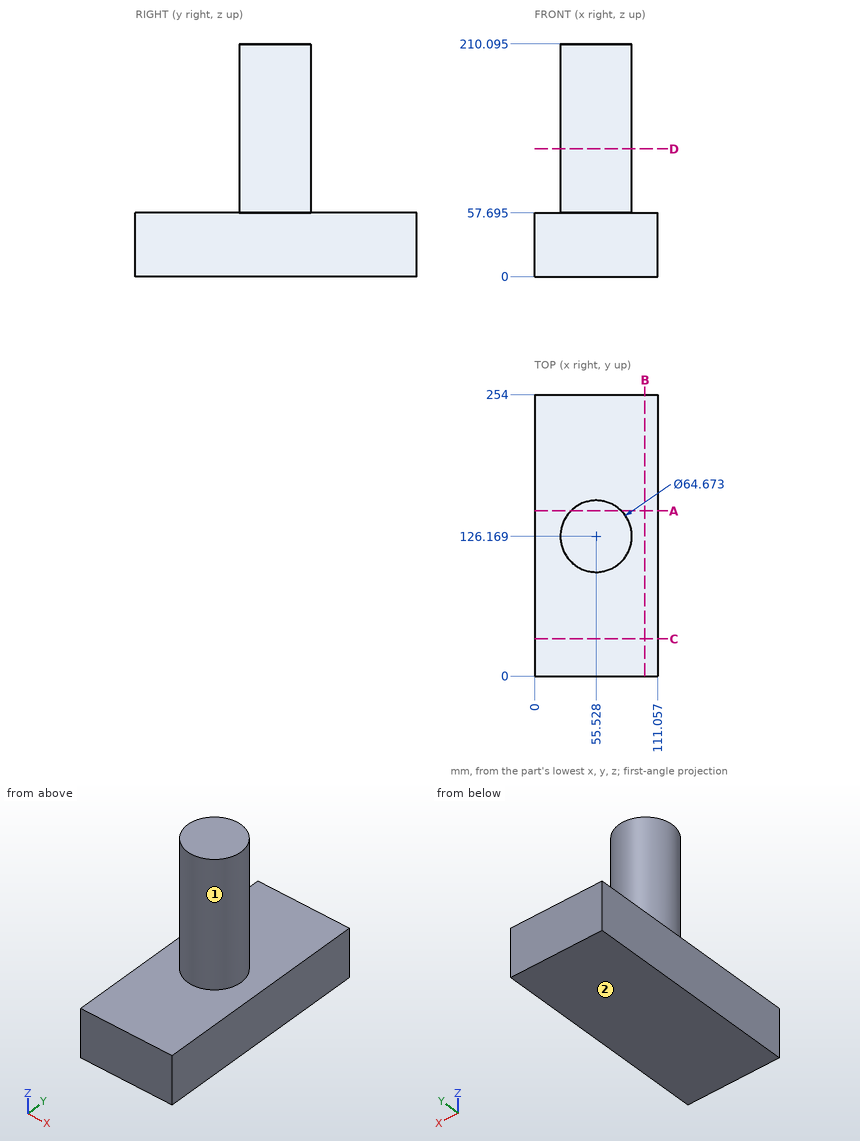
Part print with two shaded views. Sizes in mm from the minimum x, y, z corner. A direction names the side the tool comes from. Coordinates: 2 decimals unless noted, no trailing zeros. Write each loop counter-clockwise with the first axis right and the second up, starting at its lowest first coordinate (ties: lowest second). Pieces come first, ordered by that corner, then holes. Notation, with made-up numbers: M -23.5,74.5 L 28.5,74.5 A16 ccw 28.5,90.5 Z; hole C 68,9.5 d5. An arc over 180 degrees is marked long. Return JSON: item names as keys, results as strings.
Item 1: Slice it at C-C, the plane y = 33.5. Write the cut outline in (x, z) (1 decimal).
Findings below:
{"outline": "M 0,0 L 111.1,0 L 111.1,57.7 L 0,57.7 Z"}
Item 2: Slice it at A-A, the plane y = 149. Write the cut outline in (x, z) (1 decimal), and give its area (3 significant figures).
Findings below:
{"outline": "M 0,0 L 111.1,0 L 111.1,57.7 L 78.4,57.7 L 78.4,210.1 L 32.6,210.1 L 32.6,57.7 L 0,57.7 Z", "area": "13,400 mm2"}
Item 3: Which spindle directions (+Z, -Z, +X, -X, +Y, -Y) get a long thin tool onto all of the face, cutting with end or side? Do the marked faces 1 and 2. Say none if no direction does.
Findings below:
{"face 1": "+Z", "face 2": "-Z, +X, -X, +Y, -Y"}
Item 4: Probe line 1 (Y direction, x = 54, z = 60); line 2 (Z direction, x = 97.5, y = 53) (1 decimal); line 3 (X direction, y = 98.5, z = 70) (1 decimal). List the from-to ranges inside material, lowest first. Write a range as from..to.
Findings below:
{"line 1": "y = 93.87..158.47", "line 2": "z = 0..57.7", "line 3": "x = 38.8..72.3"}
Item 5: Slice it at D-D, the plane z = 115.5. Write the cut outline in (x, y) (1 decimal).
Findings below:
{"outline": "C 55.5,126.2 d64.7"}
Item 6: Drop flat-ended pins along their axis: pin 1 Ø1 at (x, z) = (74.5, 120.5) entering from -Y; pin 2 Ø12 at (x, y) = (41, 204) entering from +Z (1 decimal); pin 3 Ø5 at (x, z) = (81, 84) entering from +Y. Give the stop position or say it passes through.
Findings below:
{"pin 1": "stops at y = 99.63", "pin 2": "stops at z = 57.7", "pin 3": "stops at y = 148.93"}
Item 7: Slice it at B-B, the plane x = 99.5. Write the cut outline in (y, z) (1 decimal), and give its area (3 significant figures).
Findings below:
{"outline": "M 0,0 L 254,0 L 254,57.7 L 0,57.7 Z", "area": "14,700 mm2"}
